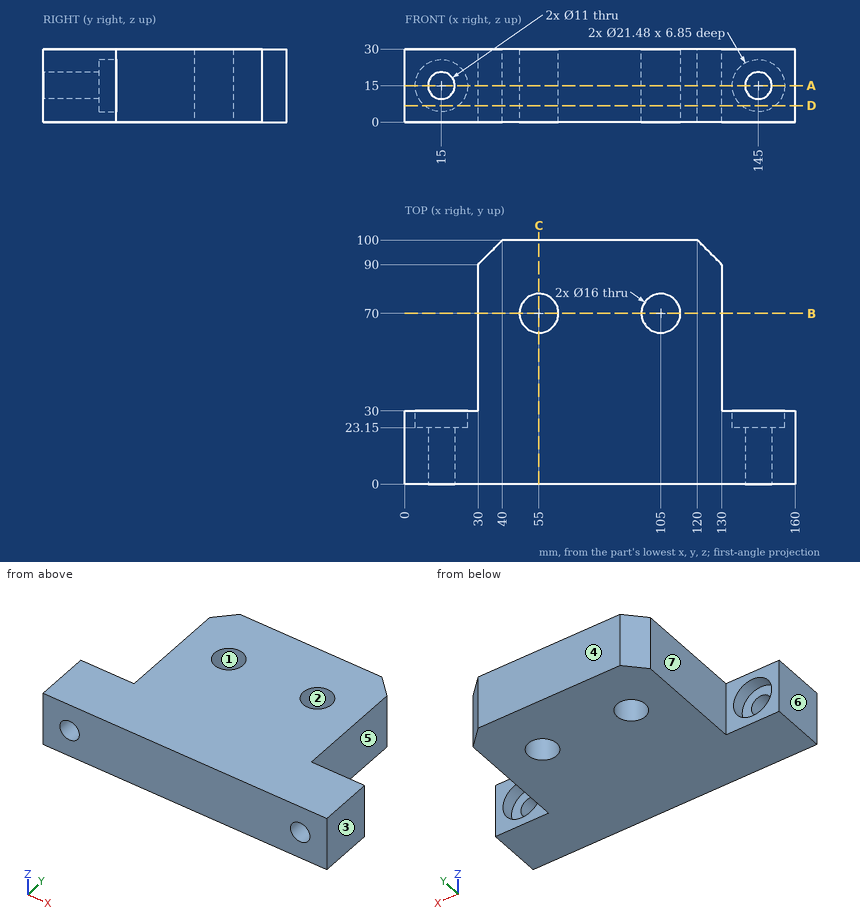
Print and shaded views of the part. All mm, measured from the part's lowest x, y and z. A direction names the side the tool comes from. Coordinates: 2 decimals unless noted, no trailing zeros. Order: outer loops, then holes, each group sorted by start corner. A loop starts at its lowest first (then second) coordinate and runs counter-clockwise, first axis right, second up. Notation, with made-up numbers: (55, 10.25) - (104, 10.25) arc R19 cw to (104, 18.25) - close; hole circle Ø11 at (42.25, 42). An arc over 180 degrees is marked (long way). Return JSON: item names as keys, results as strings. Group by question number.
Item 1: Cut at D-D (z = 6.75). List the corners of the cut face in (x, y).
Item 2: Drill centre lines: probe 1 along Y at (x, z) = (105, 14.25); probe 2 along Z at (x, y) = (145, 25); probe 3 along X at (y, z) = (5.5, 15.75). Where is each one in solid material? Low to high. Write a range as from..to.
Item 3: Cut at A-A (z = 15). List the corners of the cut face in (x, y), plus the area to 3 significant figures.
Item 4: Pin check, flat tips, straight feed: pin 1 (13 mm diameter, centred on x = 105, y = 70, fed in from +Z); pin 2 (10.5 mm diameter, centred on x = 140.5, z = 16.5, fed in from +Y); pin 3 (3 mm diameter, centred on y = 51.5, z = 14, fed in from +X); pin 4 (4 mm diameter, centred on y = 49, z = 24.5, fed in from -X). Stop position of each tip, or through.
Item 5: Cut at B-B (y = 70). List the corners of the cut face in (x, z).
Item 6: Pull direction Y, two halves, no side cores. Call the marked faces 1, 2, 3 and 4: pulls with the +Y half, pulls with the -Y half, needs draft (parallel to the pull), parting line crosses it, or undercut.
Item 7: Which spindle directions (+Z, -Z, +X, -X, +Y, -Y) get a long thin tool onto all of the face, cutting with end or side? Do the marked faces 5, 6 and 7. Say none if no direction does.
Item 8: Cut at C-C (x = 55). List the corners of the cut face in (y, z).
Check values:
{
 "1": {"outline": "(0, 0) - (160, 0) - (160, 30) - (151.88, 30) - (151.88, 23.15) - (138.12, 23.15) - (138.12, 30) - (130, 30) - (130, 90) - (120, 100) - (40, 100) - (30, 90) - (30, 30) - (21.88, 30) - (21.88, 23.15) - (8.12, 23.15) - (8.12, 30) - (0, 30) - close; hole circle Ø16 at (55, 70); hole circle Ø16 at (105, 70)"},
 "2": {"probe 1": "y = 0..62, 78..100", "probe 2": "z = 0..4.26, 25.74..30", "probe 3": "x = 0..9.55, 20.45..139.55, 150.45..160"},
 "3": {"outline": "(0, 0) - (9.5, 0) - (9.5, 23.15) - (4.26, 23.15) - (4.26, 30) - (0, 30) - close; (20.5, 0) - (139.5, 0) - (139.5, 23.15) - (134.26, 23.15) - (134.26, 30) - (130, 30) - (130, 90) - (120, 100) - (40, 100) - (30, 90) - (30, 30) - (25.74, 30) - (25.74, 23.15) - (20.5, 23.15) - close; (150.5, 0) - (160, 0) - (160, 30) - (155.74, 30) - (155.74, 23.15) - (150.5, 23.15) - close; hole circle Ø16 at (55, 70); hole circle Ø16 at (105, 70)", "area": "10,500 mm2"},
 "4": {"pin 1": "passes through", "pin 2": "stops at y = 23.15", "pin 3": "stops at x = 130", "pin 4": "stops at x = 30"},
 "5": {"outline": "(30, 0) - (47, 0) - (47, 30) - (30, 30) - close; (63, 0) - (97, 0) - (97, 30) - (63, 30) - close; (113, 0) - (130, 0) - (130, 30) - (113, 30) - close"},
 "6": {"face 1": "undercut", "face 2": "undercut", "face 3": "needs draft", "face 4": "pulls with the +Y half"},
 "7": {"face 5": "+Z, -Z, +X, +Y", "face 6": "+Z, -Z, -X, +Y, -Y", "face 7": "+Z, -Z, -X, +Y"},
 "8": {"outline": "(0, 0) - (62, 0) - (62, 30) - (0, 30) - close; (78, 0) - (100, 0) - (100, 30) - (78, 30) - close"}
}
